```python
from build123d import *

# Parameters (mm, degrees)
F1_DEPTH    = 1
F2_R        = 1.515
F3_DEPTH    = 0.86
F4_R        = 1.515
F5_DEPTH    = 0.86
F6_DEPTH    = 0.6
F8_DEPTH    = 0.8
F9_T1_DEPTH = 10.5393920142
F9_T3_DEPTH = 11
F10_R       = 1
F11_R       = 0.49999
F12_R       = 0.5


# Not quite as in the source:
# - a fillet or chamfer that OpenCascade refuses, or shapes differently, is made with other operations: its cross-section is extruded or revolved along the edge and cut away or added
# - a fillet or chamfer is up to 0.001 mm smaller than in the source, because OpenCascade refuses the exact size


with BuildPart() as f1:
    # F0 (on Top) → F1 (new body)
    with BuildSketch(Plane.XY):
        Polygon((0, 1.4), (0, 0), (7, 0), (7, 4), (0, 4), (0, 2.6), (0, 2), align=None)
        Polygon((-1, 1.4), (0, 1.4), (0, 2), (0, 2.6), (-1, 2.6), align=None)
    extrude(amount=F1_DEPTH)

    # F2 (on face) → F3 (cut)
    with BuildSketch(Plane.XY.offset(1)):
        with Locations((5, 2)):
            Circle(F2_R)
    extrude(amount=-F3_DEPTH, mode=Mode.SUBTRACT)

    # F4 (on face) → F5 (cut)
    with BuildSketch(Plane.XY.offset(1)):
        with Locations((1.99, 2)):
            Circle(F4_R)
    extrude(amount=-F5_DEPTH, mode=Mode.SUBTRACT)

    # F4 (on face) → F6 (cut)
    with BuildSketch(Plane.XY.offset(1)):
        with Locations((1.99, 2)):
            Circle(F4_R)
    extrude(amount=-F6_DEPTH, mode=Mode.SUBTRACT)

    # F7 (on face) → F8 (cut)
    with BuildSketch(Plane.XY.offset(1)):
        Polygon((-1, 2.5), (-1, 2), (-1, 1.5), (0, 1.5), (0, 2.5), align=None)
    extrude(amount=-F8_DEPTH, mode=Mode.SUBTRACT)

    # F9: fillet of radius 2 on 4 edges, made by hand

    # F9_s2 → F9_t1 (cut)
    with BuildSketch(Plane.XY.offset(-4.7696960071)):
        with BuildLine():
            ThreePointArc((1.9078784028, 4), (0.7246624462, 3.6124515497), (0, 2.6))
            Line((0, 2.6), (-0.0381575681, 2.612))
            ThreePointArc((-0.0381575681, 2.612), (-0.04, 3.3), (-0.04, 4))
            Line((-0.04, 4), (0, 4.04))
            Line((0, 4.04), (1.9078784028, 4.04))
            Line((1.9078784028, 4.04), (1.9078784028, 4))
        make_face()
        with BuildLine():
            ThreePointArc((0, 1.4), (0.7246624462, 0.3875484503), (1.9078784028, 0))
            Line((1.9078784028, 0), (1.9078784028, -0.04))
            Line((1.9078784028, -0.04), (0, -0.04))
            Line((0, -0.04), (-0.04, 0))
            ThreePointArc((-0.04, 0), (-0.04, 0.7), (-0.0381575681, 1.388))
            Line((-0.0381575681, 1.388), (0, 1.4))
        make_face()
    extrude(amount=F9_T1_DEPTH, mode=Mode.SUBTRACT)

    # F9_s4 → F9_t3 (cut)
    with BuildSketch(Plane.XY.offset(-5)):
        with BuildLine():
            ThreePointArc((7, 2), (6.4142135624, 3.4142135624), (5, 4))
            Line((5, 4), (5, 4.04))
            Line((5, 4.04), (7.04, 4.04))
            Line((7.04, 4.04), (7.04, 2))
            Line((7.04, 2), (7, 2))
        make_face()
        with BuildLine():
            ThreePointArc((5, 0), (6.4142135624, 0.5857864376), (7, 2))
            Line((7, 2), (7.04, 2))
            Line((7.04, 2), (7.04, -0.04))
            Line((7.04, -0.04), (5, -0.04))
            Line((5, -0.04), (5, 0))
        make_face()
    extrude(amount=F9_T3_DEPTH, mode=Mode.SUBTRACT)

    # F10
    f10_edges = [f1.edges().sort_by_distance(p)[0] for p in [
        (0, 1.4, 0.5),
        (0, 2.6, 0.5),
    ]]
    fillet(f10_edges, radius=F10_R)

    # F11 (radius 0.5 in the source; OpenCascade refuses exactly that, so slightly less here)
    f11_edges = [f1.edges().sort_by_distance(p)[0] for p in [
        (-0.5, 2.5, 0.2),
        (-0.5, 1.5, 0.2),
        (0, 1.5, 0.6),
        (0, 2.5, 0.6),
        (0, 2, 0.2),
    ]]
    fillet(f11_edges, radius=F11_R)

    # F12
    f12_edges = [f1.edges().sort_by_distance(p)[0] for p in [
        (3.453939, 0, 0),
        (6.414214, 0.585786, 0),
    ]]
    fillet(f12_edges, radius=F12_R)


solid = f1.part
```
Can you work these out from the model? Positions are in its coordinate system, mm. A direction names the side the tool comes from. Give positions to 0.01 mm unless a question says otherwise; leave off trailing zeros. Loops run counter-clockwise (first coordinate to the right, second up) from the corner with the lowest first, then second, coordinate; pieces in that order, holes last. Notation, with made-up numbers: M 43,66 L 77,66 A32 ccw 77,102 Z; hole C -38,-39 d8. An arc over 180 degrees is marked long. Answer in a Markdown table with one row per item.
1. If I drill on line 1 along X through (y, z) = (0.85, 0.85); line 2 along X through (y, z) = (1, 0.2); line 3 along Y through (x, z) = (1.99, 0.7) (3 decimals), over which ranges is the centre line in solid material (lowest first)?
Taken from the geometry:
| item | result |
|---|---|
| line 1 | x = 0.27 to 1, 2.98 to 4.01, 5.99 to 6.64 |
| line 2 | x = 0.29 to 0.85, 3.13 to 3.86, 6.14 to 6.62 |
| line 3 | y = 0 to 0.485, 3.515 to 4 |
2. Suppose I cut it at A-A on x = 1.99. Write out the boundary of the cut face in (y, z) (3 decimals), plus the area to 3 significant figures.
Taken from the geometry:
| item | result |
|---|---|
| outline | M 0,0.5 A0.5 ccw 0.5,0 L 3.5,0 A0.5 ccw 4,0.5 L 4,1 L 3.515,1 L 3.515,0.14 L 0.485,0.14 L 0.485,1 L 0,1 Z |
| area | 1.29 mm² |
3. For pin 1 Ø1.5 at (x, y) = (6, 2) entering from +Z, with a flat end and sliding along its axis, tell me the tip position at first contact or that it passes through.
Taken from the geometry:
| item | result |
|---|---|
| pin 1 | stops at z = 1 |
4. Thinking about a two-plate mould opening in Y: for faces 1 (the cylindrical face through (0.929, 0.256, 0.747)), 2 (the flat face through (3.5, 1.4, 0)), 3 (the cylindrical face through (0.476, 2.064, 0.576)), which applies, released by +Y, released by -Y, zero draft, split by the parting line, or undercut?
Taken from the geometry:
| item | result |
|---|---|
| face 1 | released by -Y |
| face 2 | zero draft |
| face 3 | undercut |
5. Suppose I cut it at B-B on x = 4.75. Write out the boundary of the cut face in (y, z).
Taken from the geometry:
| item | result |
|---|---|
| outline | M 0,0.5 A0.5 ccw 0.5,0 L 3.5,0 A0.5 ccw 4,0.5 L 4,1 L 3.49,1 L 3.49,0.14 L 0.51,0.14 L 0.51,1 L 0,1 Z |
6. Which directions (+Z, -Z, +X, -X, +Y, -Y) give clear straight access to the entire face, cutting with the end or side of a thin tool? Please do faces 4 (the flat face through (3.6, 3, 1)), 5 (the cylindrical face through (6.514, 1.936, 0.576)).
Taken from the geometry:
| item | result |
|---|---|
| face 4 | +Z, +X, -X, +Y, -Y |
| face 5 | +Z |
